Can you work these out from the model? Positions are in its coordinate system, mm. Face numbers are marked on the shaded views. Coordinates: 2 decimals unless noted, no trailing zeros. Loops run counter-clockwise (first coordinate to the right, second up) from the corner with the lowest first, then second, coordinate; pieces in that order, holes last.
```python
from build123d import *

# Parameters (mm, degrees)
SKETCH_1_R          = 5
EXTRUDE_1_DEPTH     = 20
CHAMFER_1_SIZE      = 10
CHAMFER_1_SIZE2     = 7.191291792
SKETCH_2_R          = 5
CUT_EXTRUDE_1_DEPTH = 10


with BuildPart() as part:
    # 草图1 → 凸台-拉伸1 (new body)
    with BuildSketch(Plane.XY):
        Polygon((-58.954112629, -2.007906554), (-58.954112629, -7.007906554), (-8.954112629, -7.007906554), (-8.954112629, -2.007906554), (71.045887371, 52.992093446), (-28.954112629, 52.992093446), align=None)
        with Locations((45.756585656, 44.992093446)):
            Circle(SKETCH_1_R, mode=Mode.SUBTRACT)
    extrude(amount=EXTRUDE_1_DEPTH)

    # 倒角1
    chamfer_1_edges = [part.edges().sort_by_distance(p)[0] for p in [
        (71.045887371, 52.992093446, 10),
    ]]
    chamfer_1_side = [part.faces().sort_by_distance(p)[0] for p in [
        (31.045887371, 25.492093446, 10),
    ]]
    chamfer(chamfer_1_edges, length=CHAMFER_1_SIZE, length2=CHAMFER_1_SIZE2, reference=chamfer_1_side[0])

    # 草图2 → 切除-拉伸1 (cut)
    with BuildSketch(Plane.XZ.offset(7.007906554)):
        with Locations((-23.954112629, 10)):
            Circle(SKETCH_2_R)
    extrude(amount=-CUT_EXTRUDE_1_DEPTH, mode=Mode.SUBTRACT)


solid = part.part
```
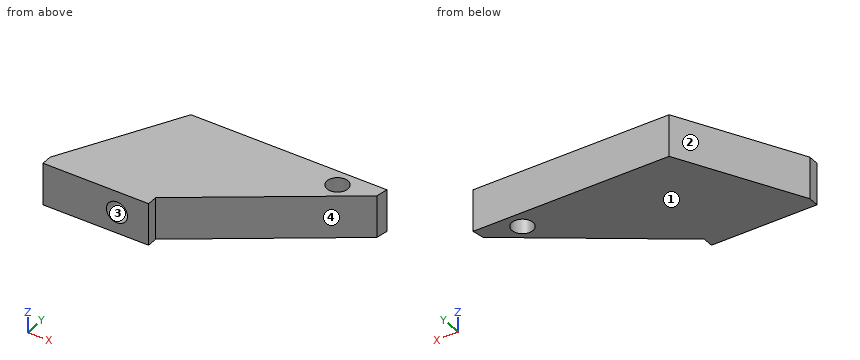
(1) I'm going to push flat-ended pins straight in: pin 1 (6 mm diameter, centred on y = 3, z = 3, fed in from +X); pin 2 (2 mm diameter, centred on x = -46.5, z = 9, fed in from +Y); pin 3 (8 mm diameter, centred on y = 34, z = 9.5, fed in from +X). Where does each tip first touch, or does it pass through?
Check values:
pin 1: stops at x = 2.69
pin 2: stops at y = 22.66
pin 3: stops at x = 49.24
(2) I want a section at B-B on x = -24. Write out the boundary of the cut face in (y, z).
Check values:
outline: (-7.01, 0) - (52.99, 0) - (52.99, 20) - (-7.01, 20) - (-7.01, 15) - (2.99, 15) - (2.99, 5) - (-7.01, 5) - close
(3) I want a section at D-D on y = 15.5. Write out the boundary of the cut face in (x, z).
Check values:
outline: (-49.4, 0) - (16.51, 0) - (16.51, 20) - (-49.4, 20) - close
(4) If I drill on probe 1 along Z at (x, y) = (-21.5, -1.5); probe 2 along X at (y, z) = (44.5, 17); probe 3 along Y at (x, z) = (52.5, 18.75), over which ranges is the centre line in solid material (lowest first)?
Check values:
probe 1: z = 0 to 5.64, 14.36 to 20
probe 2: x = -33.59 to 40.78, 50.73 to 58.69
probe 3: y = 40.24 to 52.99
(5) I want a section at C-C on z = 17.25. Write out the boundary of the cut face in (x, y), then the cut area to 3 significant figures.
Check values:
outline: (-58.95, -7.01) - (-8.95, -7.01) - (-8.95, -2.01) - (62.81, 47.33) - (63.85, 52.99) - (-28.95, 52.99) - (-58.95, -2.01) - close; hole circle Ø10 at (45.76, 44.99)
area: 4,280 mm2
(6) If we mould it in two halves opening along X, with no side actions, what happens to the marked faces 1, 2, 3 and 4? For each: released by +X, released by -X, zero draft, split by the parting line, or undercut.
Check values:
face 1: zero draft
face 2: released by -X
face 3: undercut
face 4: released by +X
(7) I want a section at A-A on z = 7. Write out the boundary of the cut face in (x, y), then the cut area to 3 significant figures.
Check values:
outline: (-58.95, -7.01) - (-27.95, -7.01) - (-27.95, 2.99) - (-19.95, 2.99) - (-19.95, -7.01) - (-8.95, -7.01) - (-8.95, -2.01) - (62.81, 47.33) - (63.85, 52.99) - (-28.95, 52.99) - (-58.95, -2.01) - close; hole circle Ø10 at (45.76, 44.99)
area: 4,200 mm2
